```python
from build123d import *

# Parameters (mm, degrees)
SKETCH4_R                = 4.7244
STOCK_DEPTH              = 4.4196
SKETCH7_R                = 7.8994
CV_GEAR_WELL_DEPTH       = 4.0132
SKETCH8_R                = 2.2987
IDLER_GEAR_WELL_DEPTH    = 4.2926
SKETCH9_R                = 4.4196
SKETCH9_R_2              = 1.27
OUTDRIVE_GEAR_WELL_DEPTH = 4.4196


with BuildPart() as part:
    # Sketch4 → Stock (new body)
    with BuildSketch(Plane.XY):
        with BuildLine():
            Line((17.301339891, -8.805936455), (17.27639382, -11.980838452))
            ThreePointArc((17.27639382, -11.980838452), (18.188661549, -14.233139719), (20.426349746, -15.180686521))
            Line((20.426349746, -15.180686521), (45.825565725, -15.380255093))
            ThreePointArc((45.825565725, -15.380255093), (48.077866993, -14.467987364), (49.025413794, -12.230299167))
            Line((49.025413794, -12.230299167), (49.224982366, 13.168916813))
            ThreePointArc((49.224982366, 13.168916813), (48.312714637, 15.42121808), (46.07502644, 16.368764882))
            Line((46.07502644, 16.368764882), (20.675810461, 16.568333454))
            ThreePointArc((20.675810461, 16.568333454), (18.423509193, 15.656065724), (17.475962392, 13.418377528))
            Line((17.475962392, 13.418377528), (17.45101632, 10.24347553))
            Line((17.45101632, 10.24347553), (-20.178385282, 10.539140008))
            Line((-20.178385282, 10.539140008), (-20.16555609, 12.171919255))
            ThreePointArc((-20.16555609, 12.171919255), (-21.077823819, 14.424220522), (-23.315512016, 15.371767324))
            Line((-23.315512016, 15.371767324), (-32.840218009, 15.446605538))
            ThreePointArc((-32.840218009, 15.446605538), (-35.092519276, 14.534337809), (-36.040066078, 12.296649612))
            Line((-36.040066078, 12.296649612), (-36.114904292, 2.77194362))
            ThreePointArc((-36.114904292, 2.77194362), (-35.202636563, 0.519642353), (-32.964948366, -0.427904449))
            Line((-32.964948366, -0.427904449), (-26.932171442, -0.475305624))
            Line((-26.932171442, -0.475305624), (-26.969946706, -5.282986868))
            ThreePointArc((-26.969946706, -5.282986868), (-26.057678977, -7.535288135), (-23.81999078, -8.482834937))
            Line((-23.81999078, -8.482834937), (17.301339891, -8.805936455))
        make_face()
        with Locations((33.387081626, 0.456569756)):
            Circle(SKETCH4_R, mode=Mode.SUBTRACT)
    extrude(amount=STOCK_DEPTH)

    # Sketch7 → CV Gear Well (cut)
    with BuildSketch(Plane(origin=(0, 0, 0), x_dir=(-1, 0, 0), z_dir=(0, 0, -1))):
        with Locations((-33.387081626, 0.456569756)):
            Circle(SKETCH7_R)
    extrude(amount=-CV_GEAR_WELL_DEPTH, mode=Mode.SUBTRACT)

    # Sketch8 → Idler Gear Well (cut)
    with BuildSketch(Plane(origin=(0, 0, 0), x_dir=(-1, 0, 0), z_dir=(0, 0, -1))):
        with Locations((-12.305081626, 0.456569756)):
            Circle(SKETCH8_R)
        with Locations((2.477718374, 0.456569756)):
            Circle(SKETCH8_R)
        with Locations((17.260518374, 0.456569756)):
            Circle(SKETCH8_R)
    extrude(amount=-IDLER_GEAR_WELL_DEPTH, mode=Mode.SUBTRACT)

    # Sketch9 → Outdrive Gear Well (cut)
    with BuildSketch(Plane(origin=(0, 0, 0), x_dir=(-1, 0, 0), z_dir=(0, 0, -1))):
        with Locations((28.055981517, 6.851899403)):
            Circle(SKETCH9_R)
        with Locations((-46.050080369, 13.193862884)):
            Circle(SKETCH9_R_2)
        with Locations((-20.650864389, 13.393431456)):
            Circle(SKETCH9_R_2)
        with Locations((-20.451295817, -12.005784524)):
            Circle(SKETCH9_R_2)
        with Locations((23.795044709, -5.307932939)):
            Circle(SKETCH9_R_2)
    extrude(amount=-OUTDRIVE_GEAR_WELL_DEPTH, mode=Mode.SUBTRACT)


solid = part.part
```
Design review of the part built by this model. Coordinates are the model's own, in mm. A direction names the side the tool comes from. Round coordinates to 2 decimals unless told otherwise and drop trailing zeros. Write each loop counter-clockwise with the first axis right and the second up, starting at its lowest first coordinate (ties: lowest second). Pieces come first, ordered by that corner, then holes.
Item 1: The part is to be moulded in two halves that separate along Y. For faces 3 (the cylindrical face through (18.45, 15.68, 2.18)), 4 (the cylindrical face through (46.325, 11.954, 2.179)), 5 (the flat face through (6, 1, 4.42)), say which applies: +Y half, -Y half, draft (parallel to the pull), parting line (faces both ways), or undercut.
Item 2: For probe 1 along X at (y, z) = (3, 4.05); probe 2 along X at (y, z) = (-5.5, 1.3); probe 3 along X at (y, z) = (9, 3.3), list the stretches that pass through material, from the lowest coordinate up.
Item 3: We need section A-A on z = 0.9. State how many separate pieces and enclosed holes the cut face has, and give its area (3 significant figures).
Item 4: Clearance check with flat-ended pins moving along their axes: pin 1 Ø1 at (x, z) = (-22.5, 2.5) entering from -Y; pin 2 Ø2 at (x, y) = (20.45, -12.01) entering from +Z; pin 3 Ø2 at (y, z) = (-2.5, 4) entering from -X; pin 4 Ø3 at (x, y) = (12.31, 0.46) entering from -Z. State where each tip first meets the part, or that it passes through.
Item 5: For faces 1 (the cylindrical face through (20.816, 14.653, 2.179)), 2 (the cylindrical face through (-4.601, -0.424, 2.116)), list the 3-axis set-ups (+Z, -Z, +X, -X, +Y, -Y) from which the entire face can be reached by the end or side of a thin tool; tool diameter is ignored.
Item 6: We need section B-B on x = 40. Write out the cut boundary in (y, z).
Returned:
1. face 3: +Y half
1. face 4: undercut
1. face 5: draft
2. probe 1: x = -36.11 to -30.22, -25.89 to 29.41, 37.37 to 49.15
2. probe 2: x = -26.96 to -25.05, -22.54 to 28.2, 38.58 to 49.08
2. probe 3: x = -36.07 to -31.92, -24.19 to 49.19
3. separate pieces: 1
3. enclosed holes: 9
3. area: 1,690 mm2
4. pin 1: stops at y = -8.5
4. pin 2: passes through
4. pin 3: stops at x = -26.96
4. pin 4: stops at z = 4.29
5. face 1: +Z, -Z
5. face 2: -Z
6. outline: (-15.33, 0) - (-3.86, 0) - (-3.86, 4.01) - (4.78, 4.01) - (4.78, 0) - (16.42, 0) - (16.42, 4.42) - (-15.33, 4.42) - close
